The model under review builds one solid part; all positions refer to its coordinate system, in mm. Round coordinates to 2 decimals unless told otherwise and drop trailing zeros. Write each loop counter-clockwise with the first axis right and the second up, starting at its lowest first coordinate (ties: lowest second). Pieces come first, ordered by that corner, then holes. Notation, with made-up numbers: (0.5, -1) - (45.5, -1) arc R14 ccw to (45.5, 24) - close; hole circle Ø4 at (37.5, 56.5). An arc over 180 degrees is marked (long way). One line per question, with ' | ' between items. Start each with the question number.
Autodesk Inventor part; units mm, degrees
ref_plane "YZ Plane" through (0, 0, 0) normal (1, 0, 0) x (0, 1, 0)
ref_plane "XZ Plane" through (0, 0, 0) normal (0, 1, 0) x (-1, 0, 0)
ref_plane "XY Plane" through (0, 0, 0) normal (0, 0, 1) x (1, 0, 0)
sketch "Base" plane through (0, 0, 0) normal (1, 0, 0) x (0, 1, 0)
  line L0 (3, -26) -> (0, -26)
  line L1 (3, -26) -> (12, -7.9488)
  line L2 (12, -7.9488) -> (12, -2.1159)
  line L3 (12, -2.1159) -> (0, 0)
  line L4 (0, -26) -> (0, 0)
  dimension "d0" = 12
  dimension "d1" = 80
  dimension "d2" = 26.5
  dimension "d3" = 26
  dimension "d4" = 3
extrude "BaseFeature" add sketch "Base" along normal blind 3
fillet "BaseFilletsFeature" radius 1.5 1 edges at (1.5, 0, 0)
sketch "BaseHoles" plane through (0, 0, 0) normal (-1, 0, 0) x (0, 0, 1)
  line L0 (-26, 3) -> (-0.529, 3) construction
  line L1 (-0.3104, 1.7605) -> (-2.1159, 12) construction
  circle A0 centre (-18.029, 3) radius 1.75
  circle A1 centre (-4.029, 3) radius 1.75
  circle A2 centre (-18.029, 3) radius 7 construction
  circle A3 centre (-4.029, 3) radius 7 construction
  line L2 (-4.029, 3) -> (-7.0452, 11.7599) construction
  line L3 (-2.1159, 12) -> (-0.3104, 1.7605)
  circle A4 centre (-6.0949, 9) radius 1.75
  line L4 (-1.7876, 0) -> (-26, 0)
  line L5 (-7.9488, 12) -> (-2.1159, 12)
  dimension "d9" = 3.5
  dimension "d12" = 3.5
  dimension "d14" = 14
  dimension "d22" = 14
  dimension "d23" = 3
  dimension "d24" = 3
  dimension "d25" = 9
hole "BaseHolesFeature" at (0, 3, -18.029) at (0, 3, -4.029) at (0, 9, -6.0949) direction (1, 0, 0) diameter 2.5 end through all
equation "\"d24\" = d23"
properties part number "VibroKnuckle"
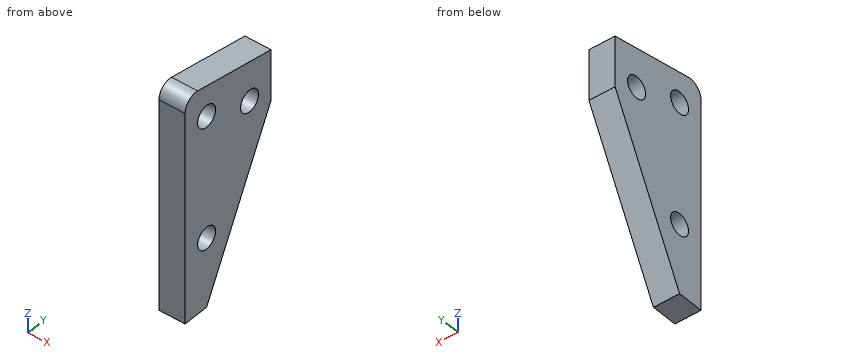
1. Wall thickness on line 1 along Z through (x, y) = (2, 4); line 2 along Y through (x, z) = (0.4, -6); line 3 along Y through (x, z) = (0.45, -18.75): over which ranges is each line inside the solid? List them lowest first. Write a range as [from, to].
2. Clearance check with flat-ended pins moving along their axes: P1, Ø1, axis at x = 2, z = -20.5, coming from the +Y side; P2, Ø1, axis at x = 1, z = -16, coming from the +Y side. State where each tip first meets the part, or that it passes through.
3. Add section D-D, the plane y = 9. Write out the cut boundary in (x, z), then the cut area to 3 significant figures.
4. Add section B-B, the plane y = 2.75. Write out the cut boundary in (x, z).
5. Add section C-C, the plane z = -5.75. Write out the cut boundary in (x, y).
6. Add section A-A, the plane x = 0.5. Write out the cut boundary in (y, z).
Geometry check:
1) line 1: z = [-23.99, -18.78], [-17.28, -4.78], [-3.28, -0.71] | line 2: y = [0, 7.75], [10.25, 12] | line 3: y = [0, 1.98], [4.02, 6.61]
2) P1: stops at y = 5.99 | P2: stops at y = 8.24
3) outline: (0, -13.97) - (3, -13.97) - (3, -7.34) - (0, -7.34) - close; (0, -4.84) - (3, -4.84) - (3, -1.59) - (0, -1.59) - close | area: 29.6 mm2
4) outline: (0, -26) - (3, -26) - (3, -19.25) - (0, -19.25) - close; (0, -16.8) - (3, -16.8) - (3, -5.25) - (0, -5.25) - close; (0, -2.8) - (3, -2.8) - (3, -0.48) - (0, -0.48) - close
5) outline: (0, 0) - (3, 0) - (3, 7.8) - (0, 7.8) - close; (0, 10.2) - (3, 10.2) - (3, 12) - (0, 12) - close
6) outline: (0, -26) - (3, -26) - (12, -7.95) - (12, -2.12) - (1.76, -0.31) arc R1.5 ccw to (0, -1.79) - close; hole circle Ø2.5 at (3, -18.03); hole circle Ø2.5 at (3, -4.03); hole circle Ø2.5 at (9, -6.09)
